Answer from the drawing. Dimensions are ordinates in mm from the lowest x, y and z of the part. Coordinates: 2 decimals unless noted, no trailing zeros. Order: outer loops, then holes, each group sorted by start corner. A loop starts at its lowest first (then second) coordinate and runs counter-clockwise, first axis right, second up.
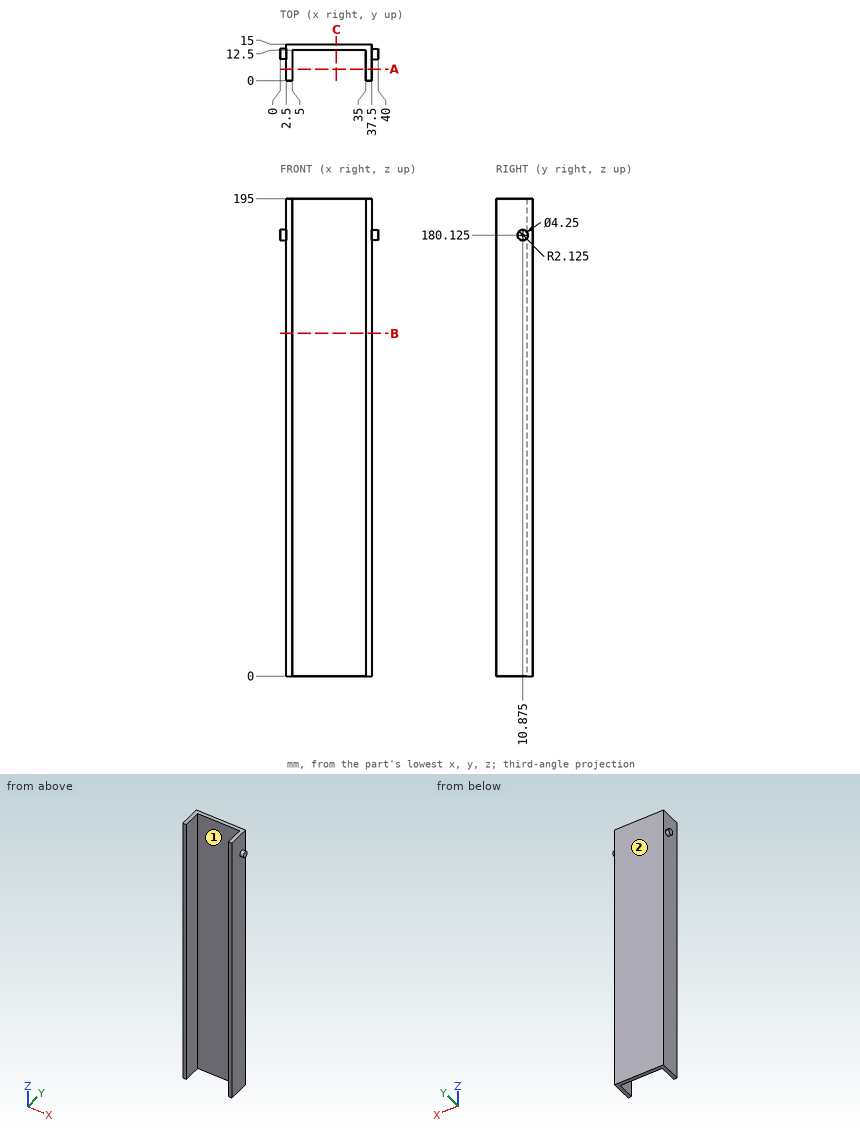
1) Section A-A (y = 4.75) is taken. Give the vertices of the cut face in (x, z), then the cut area to 3 significant figures.
2) Consider L1, parallel to X at y = 4.5, z = 32.5; L2, parallel to Y at x = 30, z = 138; L3, parallel to X at y = 13, z = 144.5. Determine where each line is inside the solid, lowest interval first.
3) Each of these flat-tipped pins is pushed along its axis until it touches: P1, Ø8, axis at y = 3, z = 27.5, coming from the +X side; P2, Ø9, axis at x = 25.5, z = 98.5, coming from the -Y side; P3, Ø4, axis at y = 8, z = 72, coming from the -X side. Where does it stop, or does it pass through?
4) Section B-B (z = 140) is taken. Give the vertices of the cut face in (x, y), then the cut area to 3 significant figures.
5) Determine the mould class of the marked faces 1 and 2 for opening direction X: released by +X, released by -X, zero draft, split by the parting line, or undercut.
6) Section C-C (x = 23) is taken. Give the vertices of the cut face in (y, z), then the cut area to 4 significant figures.
Filled sheet:
1. outline: (2.5, 0) - (5, 0) - (5, 195) - (2.5, 195) - close; (35, 0) - (37.5, 0) - (37.5, 195) - (35, 195) - close
1. area: 975 mm2
2. L1: x = 2.5 to 5, 35 to 37.5
2. L2: y = 12.5 to 15
2. L3: x = 2.5 to 37.5
3. P1: stops at x = 37.5
3. P2: stops at y = 12.5
3. P3: stops at x = 2.5
4. outline: (2.5, 0) - (5, 0) - (5, 12.5) - (35, 12.5) - (35, 0) - (37.5, 0) - (37.5, 15) - (2.5, 15) - close
4. area: 150 mm2
5. face 1: undercut
5. face 2: zero draft
6. outline: (12.5, 0) - (15, 0) - (15, 195) - (12.5, 195) - close
6. area: 487.5 mm2
